Job drawing, mm, ordinate dimensions from the low corner. One solid piece. A direction names the side the tool comes from. Coordinates: 2 decimals unless noted, no trailing zeros. Order: outer loops, then holes, each group sorted by start corner. A loop starts at its lowest first (then second) coordinate and runs counter-clockwise, first axis right, second up. Notation, with made-up numbers: (-32.5, 76) - (7.5, 76) arc R18 ccw to (7.5, 91) - close; hole circle Ø8 at (19.25, 25.25). An arc over 180 degrees is marked (long way). Use a Markdown table: item, result. Add a question column.
1) Wall check: L1, parallel to Z at x = 116, y = 51; L2, parallel to Z at x = 10.5, y = 83.5; L3, parallel to X at y = 9.5, z = 137. Give the ranges that are in metal, low to high. Write a range as [from, to].
2) Tool access for the marked faces 1, 2, 3 and 4: list every direction of +Z, -Z, +X, -X, +Y, -Y with a clear straight run to the whole face (end or side of a thin tool).
3) Saw through at B-B on y = 65. List the corners of the cut face in (x, z), then the cut area to 3 significant figures.
4) Drop flat-ended pins along their axis: P1, Ø20, axis at x = 11, y = 123.5, coming from the +Z side; P2, Ø20, axis at x = 113.5, y = 9, coming from the +Z side; P3, Ø6, axis at y = 110, z = 51, coming from the -X side; P4, Ø8, axis at y = 19.5, z = 132, coming from the -X side. Give the stop position or say it passes through.
5) Saw through at D-D on z = 61. List the corners of the cut face in (x, y) (1 decimal).
6) Saw through at A-A on z = 154. List the corners of the cut face in (x, y).
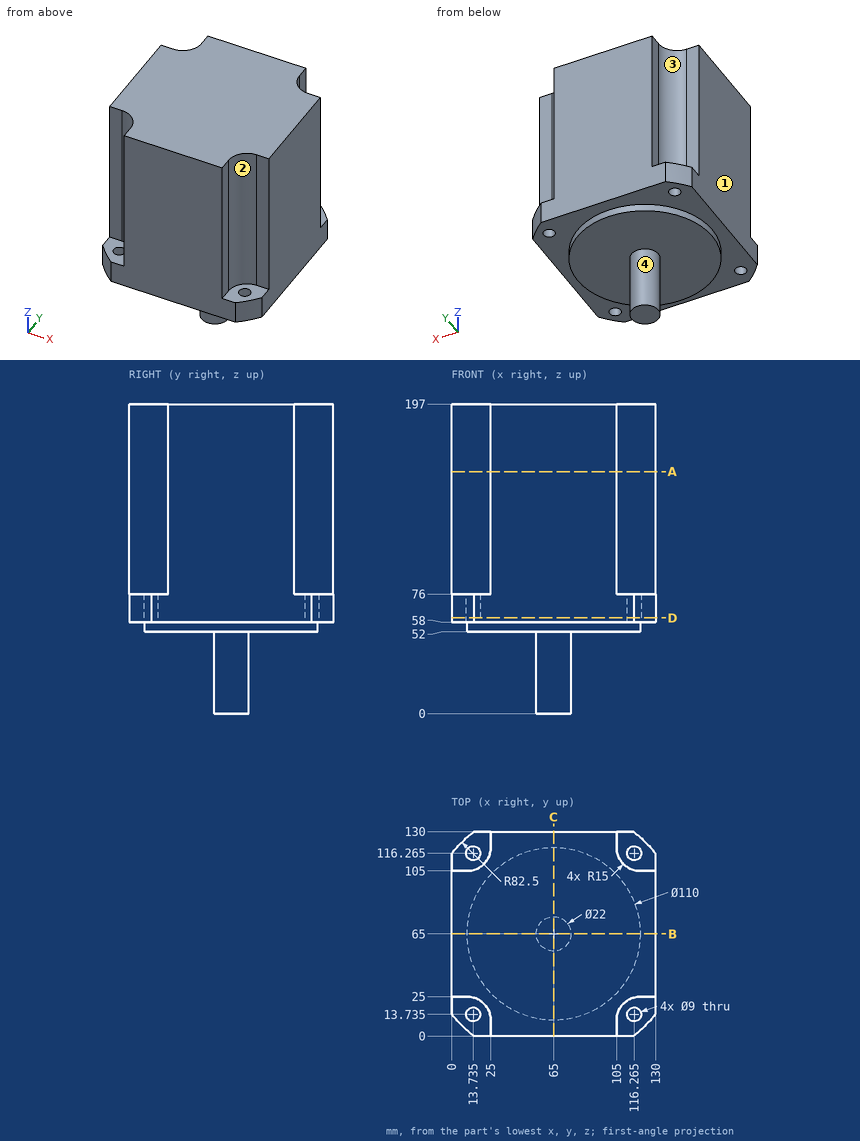
Results are:
| question | item | result |
|---|---|---|
| 1 | L1 | [52, 197] |
| 1 | L2 | [58, 197] |
| 1 | L3 | [25, 105] |
| 2 | face 1 | +Z, -Z, -X, +Y, -Y |
| 2 | face 2 | +Z, +X, -Y |
| 2 | face 3 | +Z, -X, +Y |
| 2 | face 4 | -Z |
| 3 | outline | (0, 58) - (10, 58) - (10, 52) - (54, 52) - (54, 0) - (76, 0) - (76, 52) - (120, 52) - (120, 58) - (130, 58) - (130, 197) - (0, 197) - close |
| 3 | area | 19,900 mm2 |
| 4 | P1 | z = 76 |
| 4 | P2 | z = 197 |
| 4 | P3 | x = 29.69 |
| 4 | P4 | x = 16.54 |
| 5 | outline | (0, 14.2) arc R82.5 ccw to (14.2, 0) - (115.8, 0) arc R82.5 ccw to (130, 14.2) - (130, 115.8) arc R82.5 ccw to (115.8, 130) - (14.2, 130) arc R82.5 ccw to (0, 115.8) - close; hole circle Ø9 at (13.7, 13.7); hole circle Ø9 at (13.7, 116.3); hole circle Ø9 at (116.3, 13.7); hole circle Ø9 at (116.3, 116.3) |
| 6 | outline | (0, 25) - (10, 25) arc R15 cw to (25, 10) - (25, 0) - (105, 0) - (105, 10) arc R15 cw to (120, 25) - (130, 25) - (130, 105) - (120, 105) arc R15 cw to (105, 120) - (105, 130) - (25, 130) - (25, 120) arc R15 cw to (10, 105) - (0, 105) - close |
